For this review, use the dimensioned drawing (mm, ordinates from the lowest corner) and the shaded views. A direction names the side the tool comes from. Give positions to 0.01 mm unless a question says otherwise; leave off trailing zeros. Loops run counter-clockwise (first coordinate to the right, second up) from the corner with the lowest first, then second, coordinate; pieces in that order, holes last. Notation, with made-up numbers: M -16,-23 L 40,-23 A32 cw 40,15 Z; hole C -26.5,63 d3. An arc over 180 degrees is marked long. Use a Markdown table: item, result. Add a question column.
(1) Insertion check: pin 1 Ø2 at (x, z) = (6, 9.5) entering from +Y; pin 2 Ø4 at (x, y) = (5.5, 19.5) entering from -Z; pin 3 Ø6 at (x, y) = (3.5, 4) entering from +Z. Each pin has a flat end and moves straight along its axis. Give the tip position at first contact, or say it passes through.
(2) For the marked faces 4, 5 and 6, list the 3-axis set-ups (+Z, -Z, +X, -X, +Y, -Y) from which the entire face can be reached by the end or side of a thin tool; tool diameter is ignored.
(3) For probe 1 along X at (y, z) = (11, 8.5); probe 2 along X at (y, z) = (6.25, 13.25), list the stretches that pass through material, from the lowest coordinate up.
(4) Draft analysis for pull direction Y (two halves, no side actions). For the marked faces 1, 2 and 3, state which applies: pulls with the +Y half, pulls with the -Y half, needs draft (parallel to the pull), parting line crosses it, or undercut.
(5) Add section A-A, the plane y = 11. Give the boundary of the cut face in (x, z), then the cut area to 3 significant figures.
(6) Add section D-D, the plane z = 9.5. Give the boundary of the cut face in (x, y), then the cut area to 3 significant figures.
(7) Add section C-C, the plane x = 17. Give the boundary of the cut face in (y, z).
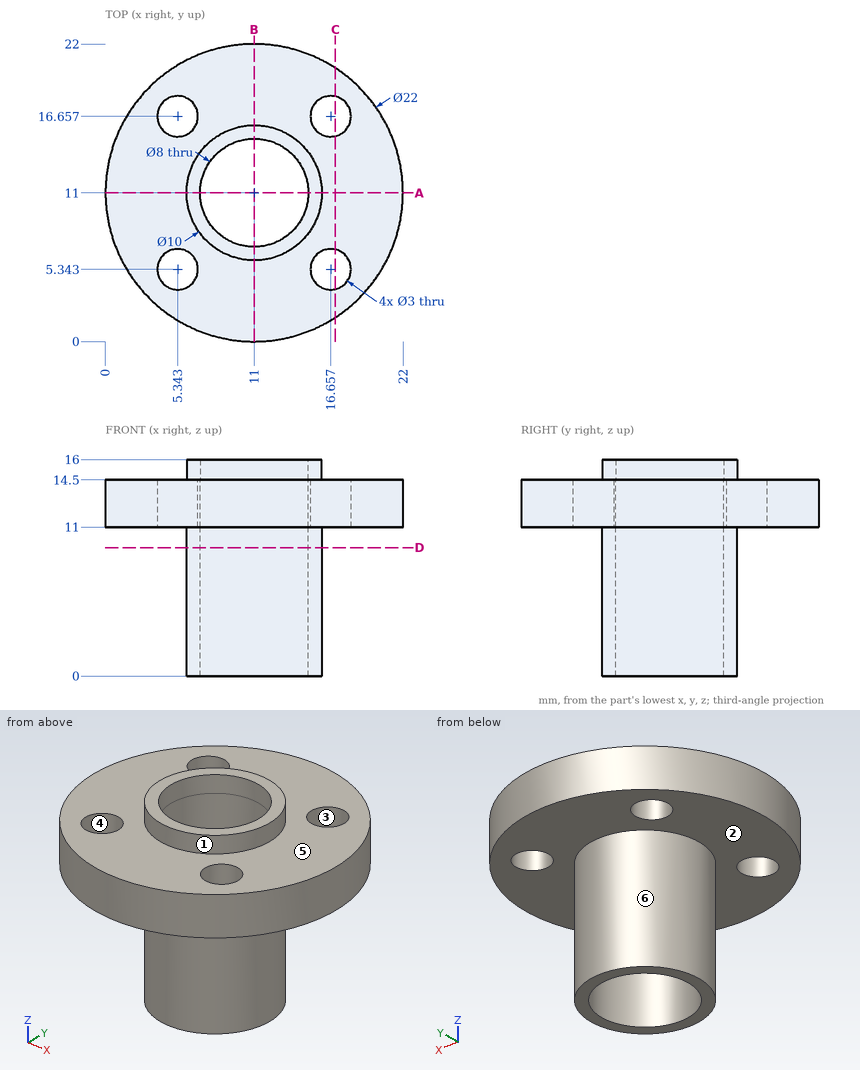
Established:
| question | item | result |
|---|---|---|
| 1 | pin 1 | y = 14 |
| 1 | pin 2 | z = 11 |
| 1 | pin 3 | z = 14.5 |
| 2 | face 4 | +Z, -Z |
| 2 | face 5 | +Z |
| 2 | face 6 | -Z |
| 3 | probe 1 | 6 to 7, 15 to 16 |
| 3 | probe 2 | 1.08 to 4.15, 6.54 to 15.46, 17.85 to 20.92 |
| 4 | face 1 | parting line crosses it |
| 4 | face 2 | needs draft |
| 4 | face 3 | undercut |
| 5 | outline | M 0,11 L 6,11 L 6,0 L 7,0 L 7,16 L 6,16 L 6,14.5 L 0,14.5 Z; M 15,0 L 16,0 L 16,11 L 22,11 L 22,14.5 L 16,14.5 L 16,16 L 15,16 Z |
| 5 | area | 74.0 mm^2 |
| 6 | outline | C 11,11 d10; hole C 11,11 d8 |
| 6 | area | 28.3 mm^2 |
| 7 | outline | M 1.78,11 L 3.88,11 L 3.88,14.5 L 1.78,14.5 Z; M 6.8,11 L 15.2,11 L 15.2,14.5 L 6.8,14.5 Z; M 18.12,11 L 20.22,11 L 20.22,14.5 L 18.12,14.5 Z |
